from build123d import *

# Parameters (mm, degrees)
TOP_VIEW_PATTERN_SKETCH_OUTSIDE_W = 104.696
TOP_VIEW_PATTERN_SKETCH_OUTSIDE_H = 104.696
TOP_VIEW_PATTERN_SKETCH_OUTSIDE_R = 6
CUT_EXTRUDE1_DEPTH                = 15
F_4_0MM_DOWEL_HOLE1_D             = 5.2


with BuildPart() as part:
    # Sketch2 → Revolve1 (revolve)
    with BuildSketch(Plane.XY):
        Polygon((-40, 0), (-17, 0), (-17, -6.8), (-15.5, -6.8), (-15.5, 0), (-13.5, 0), (-13.5, -6.8), (-12, -6.8), (-12, 2), (-40, 2), align=None)
    revolve(axis=Axis((0, 30.077146874, 0), (0, -1, 0)))

    # Top View Pattern Sketch outside → Cut-Extrude1 (cut, symmetric)
    with BuildSketch(Plane(origin=(0, 0, 0), x_dir=(1, 0, 0), z_dir=(0, 1, 0))):
        Rectangle(TOP_VIEW_PATTERN_SKETCH_OUTSIDE_W, TOP_VIEW_PATTERN_SKETCH_OUTSIDE_H)
        with BuildLine():
            Line((-10, -23.664319132), (-10, -16.522711642))
            ThreePointArc((-10, -16.522711642), (-10.475351674, -14.182143149), (-11.826086957, -12.21243904))
            ThreePointArc((-11.826086957, -12.21243904), (-14.722431864, -8.5), (-16.489325929, -4.135472212))
            ThreePointArc((-16.489325929, -4.135472212), (-17.519772084, -1.980849088), (-19.309088021, -0.398898217))
            Line((-19.309088021, -0.398898217), (-25.493901532, 3.171905528))
            ThreePointArc((-25.493901532, 3.171905528), (-28.139291346, 6.335922658), (-28.117376915, 10.460072439))
            ThreePointArc((-28.117376915, 10.460072439), (-25.980762114, 15), (-23.117376915, 19.120326477))
            ThreePointArc((-23.117376915, 19.120326477), (-19.556715651, 21.201379821), (-15.493901532, 20.492413604))
            Line((-15.493901532, 20.492413604), (-9.309088021, 16.921609859))
            ThreePointArc((-9.309088021, 16.921609859), (-7.04442041, 16.162992237), (-4.663238972, 16.347911252))
            ThreePointArc((-4.663238972, 16.347911252), (0, 17), (4.663238972, 16.347911252))
            ThreePointArc((4.663238972, 16.347911252), (7.04442041, 16.162992237), (9.309088021, 16.921609859))
            Line((9.309088021, 16.921609859), (15.493901532, 20.492413604))
            ThreePointArc((15.493901532, 20.492413604), (19.556715651, 21.201379821), (23.117376915, 19.120326477))
            ThreePointArc((23.117376915, 19.120326477), (25.980762114, 15), (28.117376915, 10.460072439))
            ThreePointArc((28.117376915, 10.460072439), (28.139291346, 6.335922658), (25.493901532, 3.171905528))
            Line((25.493901532, 3.171905528), (19.309088021, -0.398898217))
            ThreePointArc((19.309088021, -0.398898217), (17.519772084, -1.980849088), (16.489325929, -4.135472212))
            ThreePointArc((16.489325929, -4.135472212), (14.722431864, -8.5), (11.826086957, -12.21243904))
            ThreePointArc((11.826086957, -12.21243904), (10.475351674, -14.182143149), (10, -16.522711642))
            Line((10, -16.522711642), (10, -23.664319132))
            ThreePointArc((10, -23.664319132), (8.582575695, -27.537302479), (5, -29.580398915))
            ThreePointArc((5, -29.580398915), (0, -30), (-5, -29.580398915))
            ThreePointArc((-5, -29.580398915), (-8.582575695, -27.537302479), (-10, -23.664319132))
        make_face(mode=Mode.SUBTRACT)
        Circle(TOP_VIEW_PATTERN_SKETCH_OUTSIDE_R)
    extrude(amount=CUT_EXTRUDE1_DEPTH, both=True, mode=Mode.SUBTRACT)

    # Ø4.0mm Dowel Hole1 (through all)
    with Locations(Plane(origin=(0, 0, 0), x_dir=(-1, 0, 0), z_dir=(0, -1, 0))):
        with Locations((0, -23.75), (20.56810334, 11.875), (-20.56810334, 11.875)):
            Hole(F_4_0MM_DOWEL_HOLE1_D / 2)


solid = part.part
Work out the finished part from the listing and answer in its coordinate system (mm). A direction names the side the tool comes from. Give positions to 0.01 mm unless a question says otherwise; leave off trailing zeros. Write each loop counter-clockwise with the first axis right and the second up, starting at its lowest first coordinate (ties: lowest second). Pieces come first, ordered by that corner, then holes.
Q1. The part is cut by section D-D on x = 22. Give the vertices of the cut face in (y, z), and give its area (3 significant figures).
Answer:
outline: (0, -20.17) - (2, -20.17) - (2, -14.05) - (0, -14.05) - close; (0, -9.7) - (2, -9.7) - (2, -1.15) - (0, -1.15) - close
area: 29.3 mm2
Q2. For a pull along X with two mould halves and no side action, classify faces 1 (the face through (-19.368, 1.014, -9.568)), 2 (the face through (-7.078, 0.986, -16.167)), 3 (the face through (19, 0, -9)), 4 (the face through (10, 1, 20)) as released by +X, released by -X, zero draft, split by the parting line, or undercut.
Answer:
face 1: undercut
face 2: undercut
face 3: zero draft
face 4: released by +X
Q3. The part is cut by section A-A on x = 0. Give the vertices of the cut face in (y, z), and give its area (3 significant figures).
Answer:
outline: (-6.8, -17) - (2, -17) - (2, -12) - (-6.8, -12) - (-6.8, -13.5) - (0, -13.5) - (0, -15.5) - (-6.8, -15.5) - close; (-6.8, 12) - (2, 12) - (2, 21.15) - (0, 21.15) - (0, 17) - (-6.8, 17) - (-6.8, 15.5) - (0, 15.5) - (0, 13.5) - (-6.8, 13.5) - close; (0, 26.35) - (2, 26.35) - (2, 30) - (0, 30) - close
area: 76.4 mm2
Q4. Given pin 1 (1 mm diameter, centred on y = 0.5, z = 21, fed in from +X); pin 2 (1 mm diameter, centred on x = -11, y = -5, fed in from +Z); pin 3 (9 mm diameter, centred on x = 0.5, z = 24.5, fed in from -Y), each flat-ended and moving along its own axis, determine where each tip first touches the part or whether it passes through.
Answer:
pin 1: stops at x = 10
pin 2: stops at z = 13.37
pin 3: stops at y = 0
Q5. The part is cut by section B-B on z = 25. Give the vertices of the cut face in (x, y).
Answer:
outline: (-9.85, 0) - (-2.28, 0) - (-2.28, 2) - (-9.85, 2) - close; (2.28, 0) - (9.85, 0) - (9.85, 2) - (2.28, 2) - close
Q6. The part is cut by section C-C on y = -6. Give the vertices of the cut face in (x, z).
Answer:
outline: circle Ø34 at (0, 0); circle Ø27 at (0, 0); hole circle Ø31 at (0, 0); hole circle Ø24 at (0, 0)
Q7. Straight lines are drawn through the part: L1, parallel to Z at x = 0, y = -3.5; L2, parallel to Z at x = 0, y = 1.4. For each, find the intervals that lie inside material, in ascending order.
Answer:
L1: z = -17 to -15.5, -13.5 to -12, 12 to 13.5, 15.5 to 17
L2: z = -17 to -12, 12 to 21.15, 26.35 to 30
Q8. A tool of negligible diameter and unlimited length cuts with its end or side. For faces 5 (the face through (-12.44, 0.99, -18.73)), 6 (the face through (2.93, -3.45, 13.18)), 7 (the face through (28.16, 0.99, -6.39)), 8 (the face through (-10, 1, 20)), 9 (the face through (10.49, 0.99, 14.15)), from which of +Z, -Z, +X, -X, +Y, -Y can it reach the whole face along a straight path? Write none if from no direction.
Answer:
face 5: -Z, +Y, -Y
face 6: -Y
face 7: +X, +Y, -Y
face 8: +Z, -X, +Y, -Y
face 9: +Z, +X, +Y, -Y
